Part model, mm, in its own coordinate system. Face numbers are marked on the shaded views. A direction names the side the tool comes from. Round coordinates to 2 decimals unless told otherwise and drop trailing zeros. Loops run counter-clockwise (first coordinate to the right, second up) from the corner with the lowest first, then second, coordinate; pieces in that order, holes last. Notation, with made-up numbers: (50, 83.25) -> (109, 83.25) arc R14 cw to (109, 104.25) -> close; hole circle Ø4 at (59, 20.5). An arc over 180 degrees is marked (long way). Use a Markdown table: item, result. Add a question column.
Item 1: Flat gauge pins, fed straight in: pin 1 (1.5 mm diameter, centred on x = 17, z = 3.5, fed in from +Y) (3 decimals); pin 2 (1.2 mm diameter, centred on x = 33.5, z = 3, fed in from -Y); pin 3 (1 mm diameter, centred on y = 16, z = 4.5, fed in from +X). Where does each tip first touch, or does it go through?
Item 2: Cut at B-B, the plane z = 4.4. List the corners of the cut face in (x, y), plus the area to 3 significant figures.
Item 3: Cut at D-D, the plane y = 15.5. List the corners of the cut face in (x, z), plus the area to 3 significant figures.
Item 4: Probe line 1 (X direction, y = 20.25, z = 2.9); line 2 (Y direction, x = 36, z = 3.8); line 3 (X direction, y = 2.5, z = 3.05). List the from-to ranges inside material, lowest first. Write a range as [from, to].
Item 5: Cut at C-C, the plane x = 5. List the corners of the cut face in (y, z).
Item 6: Cut at A-A, the plane y = 4.25. List the corners of the cut face in (x, z).
Item 7: Which spindle directions (+Z, -Z, +X, -X, +Y, -Y) get a long thin tool onto all of the face, cutting with end or side? Do the marked faces 1 and 2. Say none if no direction does.
Autodesk Inventor part; units mm, degrees
ref_plane "YZ Plane" through (0, 0, 0) normal (1, 0, 0) x (0, 1, 0)
ref_plane "XZ Plane" through (0, 0, 0) normal (0, 1, 0) x (-1, 0, 0)
ref_plane "XY Plane" through (0, 0, 0) normal (0, 0, 1) x (1, 0, 0)
sketch "Sketch1" plane through (0, 0, 0) normal (0, 0, 1) x (1, 0, 0)
  line L0 (0, 0) -> (0, 5)
  line L1 (0, 5) -> (4.2, 5)
  line L2 (4.2, 5) -> (4.2, 0)
  line L3 (4.2, 0) -> (5.7, 0)
  line L4 (-1.5, 7.5) -> (-1.5, 0)
  line L5 (-1.5, 0) -> (0, 0)
  line L6 (40.5, 24.5) -> (40.5, 17)
  line L7 (40.5, 17) -> (39, 17)
  line L8 (39, 17) -> (39, 22)
  line L9 (39, 22) -> (34, 22)
  line L10 (34, 22) -> (34, 17)
  line L11 (34, 17) -> (32.5, 17)
  line L12 (40.5, 24.5) -> (32.5, 24.5)
  line L13 (32.5, 17) -> (32.5, 24.5)
  line L14 (-1.5, 7.5) -> (5.7, 7.5)
  line L15 (5.7, 0) -> (5.7, 7.5)
  line L16 (-1.5, 7.5) -> (32.5, 24.5)
  line L17 (5.7, 0) -> (32.5, 17)
  dimension "d0" = 17
  dimension "d1" = 5
  dimension "d2" = 4.2
  dimension "d4" = 1.5
  dimension "d5" = 1.5
  dimension "d7" = 5
  dimension "d8" = 5
  dimension "d9" = 2.5
  dimension "d10" = 2.5
  dimension "d11" = 34
extrude "Extrusion1" add sketch "Sketch1" along normal blind 6
properties part number "StrumArm"
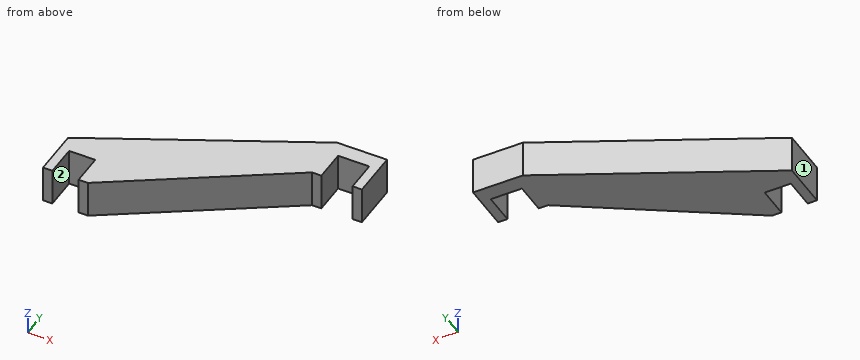
A:
| question | item | result |
|---|---|---|
| 1 | pin 1 | stops at y = 17.125 |
| 1 | pin 2 | stops at y = 17 |
| 1 | pin 3 | stops at x = 31.71 |
| 2 | outline | (-1.5, 0) -> (0, 0) -> (0, 5) -> (4.2, 5) -> (4.2, 0) -> (5.7, 0) -> (32.5, 17) -> (34, 17) -> (34, 22) -> (39, 22) -> (39, 17) -> (40.5, 17) -> (40.5, 24.5) -> (32.5, 24.5) -> (-1.5, 7.5) -> close |
| 2 | area | 330 mm^2 |
| 3 | outline | (14.5, 0) -> (30.14, 0) -> (30.14, 6) -> (14.5, 6) -> close |
| 3 | area | 93.8 mm^2 |
| 4 | line 1 | x = [24, 34], [39, 40.5] |
| 4 | line 2 | y = [22, 24.5] |
| 4 | line 3 | x = [-1.5, 0], [4.2, 9.64] |
| 5 | outline | (0, 0) -> (10.75, 0) -> (10.75, 6) -> (0, 6) -> close |
| 6 | outline | (-1.5, 0) -> (0, 0) -> (0, 6) -> (-1.5, 6) -> close; (4.2, 0) -> (12.4, 0) -> (12.4, 6) -> (4.2, 6) -> close |
| 7 | face 1 | +Z, -Z, -X, +Y, -Y |
| 7 | face 2 | +Z, -Z, -Y |
